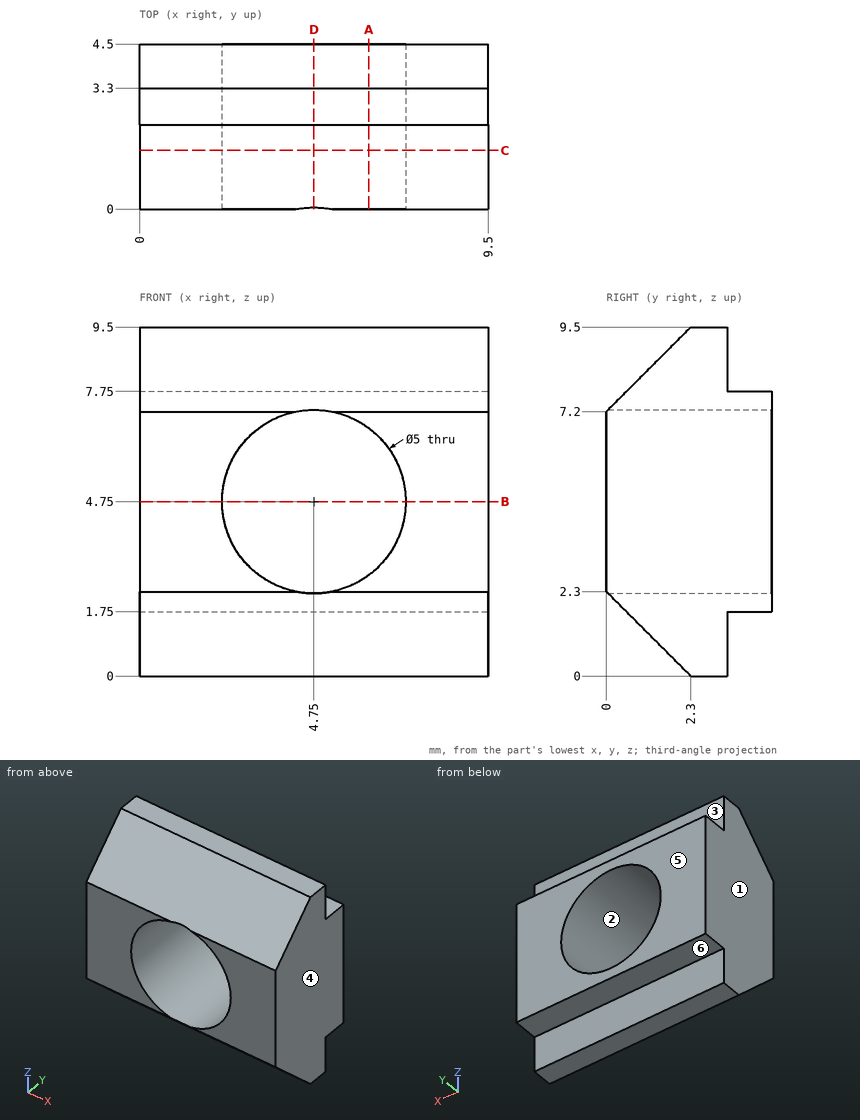
Input: dimensioned drawing with shaded views. Units: mm. Origin: part minimum x, y, z. A direction names the side the tool comes from. Coordinates: 2 decimals unless noted, no trailing zeros. Order: outer loops, then holes, each group sorted by start corner. A loop starts at its lowest first (then second) coordinate and runs counter-clockwise, first axis right, second up. Notation, with made-up numbers: (-19, -20) - (36, -20) arc R17 ccw to (36, -13) - close; hole circle Ø4 at (-9, 12.5). An arc over 180 degrees is marked (long way). Put each result on its own line as item: value.
1. Cut plane D-D on x = 4.75. Return the cut outline in (y, z).
Report:
outline: (0.05, 2.25) - (2.3, 0) - (3.3, 0) - (3.3, 1.75) - (4.5, 1.75) - (4.5, 2.25) - close; (0.05, 7.25) - (4.5, 7.25) - (4.5, 7.75) - (3.3, 7.75) - (3.3, 9.5) - (2.3, 9.5) - close
2. Cut plane A-A on x = 6.25. Return the cut outline in (y, z), then the cut area to 3 significant figures.
Report:
outline: (0, 2.3) - (2.3, 0) - (3.3, 0) - (3.3, 1.75) - (4.5, 1.75) - (4.5, 2.75) - (0, 2.75) - close; (0, 6.75) - (4.5, 6.75) - (4.5, 7.75) - (3.3, 7.75) - (3.3, 9.5) - (2.3, 9.5) - (0, 7.2) - close
area: 15.3 mm2
3. Contact query for flat-ended pins moving along their axis: pin 1 Ø2 at (x, y) = (7, 1) entering from +Z; pin 2 Ø0.6 at (x, y) = (5, 4) entering from -Z; pin 3 Ø1.3 at (x, y) = (5.5, 4) entering from +Z. Output: stop coordinate, or through.
Report:
pin 1: stops at z = 9.2
pin 2: stops at z = 1.75
pin 3: stops at z = 7.75
4. Draft query along X for the marked faces 1, 2, 3 and 4. Return one class per face: pulls with the +X half, pulls with the -X half, needs draft (parallel to the pull), parting line crosses it, or undercut.
Report:
face 1: pulls with the -X half
face 2: undercut
face 3: needs draft
face 4: pulls with the +X half
5. Cut plane B-B on z = 4.75. Return the cut outline in (x, y), then the cut area to 4 significant figures.
Report:
outline: (0, 0) - (2.25, 0) - (2.25, 4.5) - (0, 4.5) - close; (7.25, 0) - (9.5, 0) - (9.5, 4.5) - (7.25, 4.5) - close
area: 20.25 mm2
6. Line query: line 1 along X through (y, z) = (3.2, 4.75); line 2 along Z through (x, y) = (8, 3.45). Output: solid intervals per line, ascending.
Report:
line 1: x = 0 to 2.25, 7.25 to 9.5
line 2: z = 1.75 to 7.75
7. Cut plane C-C on y = 1.6. Return the cut outline in (x, z).
Report:
outline: (0, 0.7) - (9.5, 0.7) - (9.5, 8.8) - (0, 8.8) - close; hole circle Ø5 at (4.75, 4.75)
8. Reachability of the marked faces 5 and 6 from +Z, -Z, +X, -X, +Y, -Y: full face, straight path, thin tool, end or side. Return the list, or none.
Report:
face 5: +Z, -Z, +X, -X, +Y
face 6: -Z, +X, -X, +Y
